```python
from build123d import *

# Parameters (mm, degrees)
SKETCH001_W          = 70
SKETCH001_H          = 20
PAD_DEPTH            = 12.7
SKETCH012_W          = 36
SKETCH012_H          = 17
PAD001_DEPTH         = 40
POCKET_DEPTH         = 40
POCKET001_DEPTH      = 22.994766
SKETCH007_W          = 36
SKETCH007_H          = 30
PAD002_DEPTH         = 6
POCKET002_DEPTH      = 2
POCKET003_DEPTH      = 22
POCKET003_DEPTH_BACK = -100
SKETCH013_R          = 9
POCKET004_DEPTH      = 40
FILLET_R             = 1
CHAMFER_SIZE         = 2
CHAMFER001_SIZE      = 4


with BuildPart() as part:
    # Sketch001 → Pad (new body)
    with BuildSketch(Plane.XY):
        with Locations((-8, 8)):
            Rectangle(SKETCH001_W, SKETCH001_H)
    extrude(amount=PAD_DEPTH)

    # Sketch012 (on Face6 of Pad) → Pad001 (join)
    with BuildSketch(Plane.XY.offset(12.7)):
        with Locations((-8, 9.5)):
            Rectangle(SKETCH012_W, SKETCH012_H)
    extrude(amount=PAD001_DEPTH)

    # Sketch005 → Pocket (cut)
    with BuildSketch(Plane.XY.offset(52.7)):
        with BuildLine():
            ThreePointArc((-3, 5), (-8, 10), (-13, 5))
            Line((-13, -7.39), (-13, 5))
            Line((-3, -7.39), (-13, -7.39))
            Line((-3, 5), (-3, -7.39))
        make_face()
    extrude(amount=-POCKET_DEPTH, mode=Mode.SUBTRACT)

    # Sketch010 → Pocket001 (cut, through all)
    with BuildSketch(Plane(origin=(0, 20.993766, 0), x_dir=(-1, 0, 0), z_dir=(0, 1, 0))):
        with BuildLine():
            ThreePointArc((-16.5, 8.95), (-19.1, 6.35), (-16.5, 3.75))
            Line((-16.5, 3.75), (-14.5, 3.75))
            ThreePointArc((-14.5, 3.75), (-11.9, 6.35), (-14.5, 8.95))
            Line((-16.5, 8.95), (-14.5, 8.95))
        make_face()
        with BuildLine():
            ThreePointArc((30.5, 8.95), (27.9, 6.35), (30.5, 3.75))
            Line((30.5, 3.75), (32.5, 3.75))
            ThreePointArc((32.5, 3.75), (35.1, 6.35), (32.5, 8.95))
            Line((30.5, 8.95), (32.5, 8.95))
        make_face()
    extrude(amount=-POCKET001_DEPTH, mode=Mode.SUBTRACT)

    # Sketch007 → Pad002 (join)
    with BuildSketch(Plane.XY.offset(52.7)):
        with Locations((-8, 3)):
            Rectangle(SKETCH007_W, SKETCH007_H)
        with BuildLine():
            ThreePointArc((-19.25, -7), (-21, -5.25), (-22.75, -7))
            Line((-22.75, -7), (-22.75, -9))
            ThreePointArc((-22.75, -9), (-21, -10.75), (-19.25, -9))
            Line((-19.25, -7), (-19.25, -9))
        make_face(mode=Mode.SUBTRACT)
        with BuildLine():
            ThreePointArc((6.75, -7), (5, -5.25), (3.25, -7))
            Line((3.25, -7), (3.25, -9))
            ThreePointArc((3.25, -9), (5, -10.75), (6.75, -9))
            Line((6.75, -7), (6.75, -9))
        make_face(mode=Mode.SUBTRACT)
    extrude(amount=PAD002_DEPTH)

    # Sketch008 → Pocket002 (cut)
    with BuildSketch(Plane.XY.offset(56.7)):
        Polygon((5.856406, 5), (-1.071797, 17), (-14.928203, 17), (-21.856406, 5), (-14.928203, -7), (-1.071797, -7), align=None)
    extrude(amount=POCKET002_DEPTH, mode=Mode.SUBTRACT)

    # Sketch006 → Pocket003 (cut, two sides)
    with BuildSketch(Plane.XY.offset(12.7)) as pocket003_sk:
        with BuildLine():
            ThreePointArc((-3.5, 6), (-8, 10.5), (-12.5, 6))
            Line((-12.5, 6), (-12.5, 4))
            ThreePointArc((-12.5, 4), (-8, -0.5), (-3.5, 4))
            Line((-3.5, 6), (-3.5, 4))
        make_face()
    extrude(amount=-POCKET003_DEPTH, mode=Mode.SUBTRACT)
    extrude(pocket003_sk.sketch, amount=-POCKET003_DEPTH_BACK, mode=Mode.SUBTRACT)

    # Sketch013 (on Face29 of Pocket003) → Pocket004 (cut)
    with BuildSketch(Plane.XY.offset(56.7)):
        with Locations((-8, 5)):
            Circle(SKETCH013_R)
    extrude(amount=-POCKET004_DEPTH, mode=Mode.SUBTRACT)

    # Fillet
    fillet_edges = [part.edges().sort_by_distance(p)[0] for p in [
        (0.062258, 1, 34.7),
        (-16.062258, 1, 34.7),
    ]]
    fillet(fillet_edges, radius=FILLET_R)

    # Chamfer
    chamfer_edges = [part.edges().sort_by_distance(p)[0] for p in [
        (10, -12, 55.7),
        (-26, -12, 55.7),
    ]]
    chamfer(chamfer_edges, length=CHAMFER_SIZE)

    # Chamfer001
    chamfer001_edges = [part.edges().sort_by_distance(p)[0] for p in [
        (-43, 18, 6.35),
        (27, 18, 6.35),
    ]]
    chamfer(chamfer001_edges, length=CHAMFER001_SIZE)


solid = part.part
```
For this review, take the finished solid that the model builds, in its own axes (mm). A direction names the side the tool comes from. Coordinates: 2 decimals unless noted, no trailing zeros. Write each loop counter-clockwise with the first axis right and the second up, starting at its lowest first coordinate (ties: lowest second). Pieces come first, ordered by that corner, then holes. Notation, with made-up numbers: (63.5, 45) - (94.5, 45) arc R9 ccw to (94.5, 50) - close; hole circle Ø6 at (28, 18.25). An arc over 180 degrees is marked (long way). Answer in a Markdown table with one row per item. Add a question column.
Q1. We need section B-B, the plane x = -8. State the section outline as (y, z) points, and give its area (3 significant figures).
Q2. We need section A-A, the plane z = 6.35. State the section outline as (x, y) points, and give its area (3 significant figures).
Q3. Draft analysis for pull direction Z (two halves, no side actions). For faces 6 (the flat face through (2.344, -1.084, 57.686)), 7 (the flat face through (-31, 8, 3.75)), 8 (the flat face through (1, 3, 56.7)), 9 (the flat face through (-31, 8, 8.95)), state which applies: +Z half, -Z half, draft (parallel to the pull), parting line (faces both ways), or undercut.
Q4. We need section D-D, the plane y = 15.75. State the section outline as (x, z) points.
Q5. We need section C-C, the plane z = 15.5. State the section outline as (x, y) points (3 decimals), and give its area (3 significant figures).
Q6. For P1, Ø1, axis at y = -8, z = 56.5, coming from the +X side; P2, Ø10.5, axis at x = -17.5, z = 35.5, coming from the -Y side; P3, Ø1, axis at y = -7.5, z = 56, coming from the -X side; P4, Ø1.5, axis at x = -27.5, y = -4, coming from the +Z side, all flat-tipped, find the tip position at first contact; note any pin that passes through.
Q7. For probe 1 along X at (y, z) = (5, 47.5); probe 2 along X at (y, z) = (16.75, 33); probe 3 along Z at (x, y) = (-25, -9.75), list the stretches that pass through material, from the lowest coordinate up.
Q8. Tool access review of faces 1 (the flat face through (27, 6, 6)), 2 (the flat face through (-8, -2, 6)), 3 (the flat face through (5, 1, 32)), 4 (the flat face through (6.75, -8, 56)), 5 (the cylindrical face through (-3.226, 6.487, 14.728)): name each direction out of +Z, -Z, +X, -X, +Y, -Y from which nothing blocks a thin tool from reaching the whole face with its end or side.
Answer list:
| question | item | result |
|---|---|---|
| 1 | outline | (-12, 52.7) - (-4, 52.7) - (-4, 56.7) - (-7, 56.7) - (-7, 58.7) - (-12, 58.7) - close; (-2, 0) - (-0.5, 0) - (-0.5, 12.7) - (-2, 12.7) - close; (10.5, 0) - (18, 0) - (18, 58.7) - (17, 58.7) - (17, 56.7) - (14, 56.7) - (14, 16.7) - (10.5, 16.7) - close |
| 1 | area | 348 mm2 |
| 2 | outline | (-43, -2) - (-35.1, -2) - (-35.1, 18) - (-39, 18) - (-43, 14) - close; (-27.9, -2) - (11.9, -2) - (11.9, 18) - (-27.9, 18) - close; (19.1, -2) - (27, -2) - (27, 14) - (23, 18) - (19.1, 18) - close; hole (-12.5, 4) arc R4.5 ccw to (-3.5, 4) - (-3.5, 6) arc R4.5 ccw to (-12.5, 6) - close |
| 2 | area | 1,010 mm2 |
| 3 | face 6 | draft |
| 3 | face 7 | undercut |
| 3 | face 8 | +Z half |
| 3 | face 9 | undercut |
| 4 | outline | (-41.25, 0) - (25.25, 0) - (25.25, 12.7) - (10, 12.7) - (10, 58.7) - (-0.35, 58.7) - (-0.35, 56.7) - (-15.65, 56.7) - (-15.65, 58.7) - (-26, 58.7) - (-26, 12.7) - (-41.25, 12.7) - close; hole (-32.5, 3.75) - (-30.5, 3.75) arc R2.6 ccw to (-30.5, 8.95) - (-32.5, 8.95) arc R2.6 ccw to start; hole (14.5, 3.75) - (16.5, 3.75) arc R2.6 ccw to (16.5, 8.95) - (14.5, 8.95) arc R2.6 ccw to start |
| 5 | outline | (-26, 1) - (-13, 1) - (-13, 5) arc R5 cw to (-12.091, 7.875) arc R4.5 cw to (-3.909, 7.875) arc R5 cw to (-3, 5) - (-3, 1) - (10, 1) - (10, 18) - (-26, 18) - close |
| 5 | area | 529 mm2 |
| 6 | P1 | stops at x = 10 |
| 6 | P2 | stops at y = 1 |
| 6 | P3 | stops at x = -26 |
| 6 | P4 | passes through |
| 7 | probe 1 | x = -26 to -17, 1 to 10 |
| 7 | probe 2 | x = -26 to 10 |
| 7 | probe 3 | z = 52.7 to 58.7 |
| 8 | face 1 | +Z, -Z, +X, +Y, -Y |
| 8 | face 2 | -Z, +X, -X, -Y |
| 8 | face 3 | +X, -X, -Y |
| 8 | face 4 | +Z, -Z |
| 8 | face 5 | +Z, -Y |
